Input: part model. Units: mm. Frame: model coordinates. A direction names the side the tool comes from. Give positions to 0.01 mm unless a question says otherwise; leave off trailing zeros. Write each loop counter-clockwise with the first axis right and the second up, starting at its lowest first coordinate (ties: lowest second). Pieces come first, ordered by that corner, then holes. Notation, with made-up numbers: (12.5, 48.25) -> (16.5, 48.25) arc R26 cw to (16.5, 71.25) -> close; hole circle Ø2 at (-20, 16). An arc over 180 degrees is marked (long way). Answer as a JSON object with one key per item and string values. Group by question number.
from build123d import *

# Parameters (mm, degrees)
SKETCH1_R                 = 4
BOSS_EXTRUDE1_DEPTH       = 20
F_5_0MM_DOWEL_HOLE1_D     = 5
F_5_0MM_DOWEL_HOLE1_DEPTH = 6
F_5_0MM_DOWEL_HOLE1_TIP   = 1.502151548
CUT_EXTRUDE1_DEPTH        = 6
CHAMFER1_SIZE             = 0.5
CHAMFER2_SIZE             = 0.65


with BuildPart() as part:
    # Sketch1 → Boss-Extrude1 (new body)
    with BuildSketch(Plane(origin=(0, 0, 0), x_dir=(1, 0, 0), z_dir=(0, 1, 0))):
        Circle(SKETCH1_R)
    extrude(amount=BOSS_EXTRUDE1_DEPTH)

    # Ø5.0mm Dowel Hole1
    with Locations(Plane(origin=(0, 20, 0), x_dir=(1, 0, 0), z_dir=(0, 1, 0))):
        with Locations((0, 0)):
            Hole(F_5_0MM_DOWEL_HOLE1_D / 2, depth=F_5_0MM_DOWEL_HOLE1_DEPTH)
            with Locations((0, 0, -(F_5_0MM_DOWEL_HOLE1_DEPTH + F_5_0MM_DOWEL_HOLE1_TIP / 2))):  # 118° drill point
                Cone(0, F_5_0MM_DOWEL_HOLE1_D / 2, F_5_0MM_DOWEL_HOLE1_TIP, mode=Mode.SUBTRACT)

    # Sketch2 → Cut-Extrude1 (cut)
    with BuildSketch(Plane(origin=(0, 20, 0), x_dir=(1, 0, 0), z_dir=(0, 1, 0))):
        Polygon((2.886751346, 0), (1.443375673, 2.5), (-1.443375673, 2.5), (-2.886751346, 0), (-1.443375673, -2.5), (1.443375673, -2.5), align=None)
    extrude(amount=-CUT_EXTRUDE1_DEPTH, mode=Mode.SUBTRACT)

    # Chamfer1
    chamfer1_edges = [part.edges().sort_by_distance(p)[0] for p in [
        (-4, 20, 0),
    ]]
    chamfer(chamfer1_edges, length=CHAMFER1_SIZE)

    # Chamfer2
    chamfer2_edges = [part.edges().sort_by_distance(p)[0] for p in [
        (-4, 0, 0),
    ]]
    chamfer(chamfer2_edges, length=CHAMFER2_SIZE)


solid = part.part
1. Section A-A (y = 15.5). Return the cut outline in (x, z), plus the area to 3 significant figures.
2. Contact query for flat-ended pins moving along their axis: pin 1 Ø1.5 at (x, y) = (2, 16) entering from +Z; pin 2 Ø3 at (x, y) = (2, 8.5) entering from +Z; pin 3 Ø1.5 at (y, z) = (16.5, -3) entering from -X. Output: stop coordinate, or through.
3. Line query: line 1 (X direction, y = 16.5, z = -0.75); line 2 (Z direction, x = -2, y = 17.25); line 3 (Z direction, x = -1.5, y = 14.5). Output: solid intervals per line, ascending.
4. Section B-B (y = 8.75). Return the cut outline in (x, z).
5. Mould query, pull axis X, two halves, no side actions, for faces 1 (the face through (-0.867, 9.943, 3.905)), 2 (the face through (0, 0, 0)), 3 (the face through (2.155, 17.042, 1.267)), 4 (the face through (-2.175, 17.042, 1.233)). Classes: pulls with the +X half, pulls with the -X half, needs draft (parallel to the pull), parting line crosses it, or undercut.
6. Reachability of faces 5 (the face through (0, 17, -2.5)), 6 (the face through (-2, 20, 2)) from +Z, -Z, +X, -X, +Y, -Y: full face, straight path, thin tool, end or side. Return the list, or none.
7. Section C-C (y = 13). Return the cut outline in (x, z).
Working result:
{
 "1": {"outline": "circle Ø8 at (0, 0); hole (-2.89, 0) -> (-1.44, -2.5) -> (1.44, -2.5) -> (2.89, 0) -> (1.44, 2.5) -> (-1.44, 2.5) -> close", "area": "28.6 mm^2"},
 "2": {"pin 1": "stops at z = 3.8", "pin 2": "stops at z = 3.97", "pin 3": "stops at x = -3.31"},
 "3": {"line 1": "x = -3.93 to -2.45, 2.45 to 3.93", "line 2": "z = -3.46 to -1.54, 1.54 to 3.46", "line 3": "z = -3.71 to -2.4, 2.4 to 3.71"},
 "4": {"outline": "circle Ø8 at (0, 0)"},
 "5": {"face 1": "parting line crosses it", "face 2": "needs draft", "face 3": "undercut", "face 4": "undercut"},
 "6": {"face 5": "+Y", "face 6": "+Z, -Z, +X, -X, +Y"},
 "7": {"outline": "circle Ø8 at (0, 0); hole circle Ø1.67 at (0, 0)"}
}
